```python
from build123d import *

# Parameters (mm, degrees)
SKETCH1_R                = 59
EXTRUDE1_DEPTH           = 3
EXTRUDE2_DEPTH           = 3
CIRPATTERN1_COUNT        = 6
F_2_0_2_DIAMETER_HOLE1_D = 2
F_2_0_2_DIAMETER_HOLE3_D = 2
CIRPATTERN2_COUNT        = 6


with BuildPart() as part:
    # Sketch1 → Extrude1 (new, symmetric)
    with BuildSketch(Plane(origin=(0, 0, 0), x_dir=(0, 0, -1), z_dir=(1, 0, 0))):
        Circle(SKETCH1_R)
        Polygon((23.694176429, 16.590840947), (-2.521001516, 28.815179183), (-26.215177945, 12.224338236), (-23.694176429, -16.590840947), (2.521001516, -28.815179183), (26.215177945, -12.224338236), align=None, mode=Mode.SUBTRACT)
    extrude(amount=EXTRUDE1_DEPTH, both=True)

    # Sketch2 → Extrude2 (add, symmetric)
    with BuildSketch(Plane(origin=(0, 0, 0), x_dir=(0, 0, -1), z_dir=(1, 0, 0))):
        with BuildLine():
            Line((-2, 67.961805723), (-0.262709442, 61.478149092))
            ThreePointArc((-0.262709442, 61.478149092), (-0.58620663, 59.77173183), (-2.122608272, 58.961805723))
            ThreePointArc((-2.122608272, 58.961805723), (28.679663449, 51.560419941), (51.21368579, 29.294340542))
            ThreePointArc((51.21368579, 29.294340542), (36.791707484, 48.186627241), (17.927108603, 62.644803614))
            ThreePointArc((17.927108603, 62.644803614), (8.312130826, 66.609702921), (-2, 67.961805723))
        make_face()
    extrude2 = extrude(amount=EXTRUDE2_DEPTH, both=True)

    # CirPattern1: Extrude2 ×6 about axis
    cirpattern1_axis = Axis((0, 0, 0), (1, 0, 0))
    for i in range(1, CIRPATTERN1_COUNT):
        add(extrude2.rotate(cirpattern1_axis, i * 360 / CIRPATTERN1_COUNT))

    # Ø2.0 (2) Diameter Hole1 (through all)
    with Locations(Plane(origin=(3, 0, 0), x_dir=(0, 0, -1), z_dir=(1, 0, 0))):
        with Locations((-2.521001516, 28.815179183), (23.694176429, 16.590840947), (26.215177945, -12.224338236), (2.521001516, -28.815179183), (-23.694176429, -16.590840947), (-26.215177945, 12.224338236)):
            Hole(F_2_0_2_DIAMETER_HOLE1_D / 2)

    # Ø2.0 (2) Diameter Hole3 (through all)
    with Locations(Plane(origin=(3, 0, 0), x_dir=(0, 0, -1), z_dir=(1, 0, 0))):
        with Locations((6.519493728, 24.599527017)):
            f_2_0_2_diameter_hole3 = Hole(F_2_0_2_DIAMETER_HOLE3_D / 2)

    # CirPattern2: Ø2.0 (2) Diameter Hole3 ×6 about axis
    cirpattern2_axis = Axis((0, 0, 0), (1, 0, 0))
    for i in range(1, CIRPATTERN2_COUNT):
        add(f_2_0_2_diameter_hole3.rotate(cirpattern2_axis, i * 360 / CIRPATTERN2_COUNT), mode=Mode.SUBTRACT)


solid = part.part
```
Here's how the part is built. I have some questions about the finished solid (model axes, mm). A direction names the side the tool comes from. Round coordinates to 2 decimals unless told otherwise and drop trailing zeros. Order: outer loops, then holes, each group sorted by start corner. A loop starts at its lowest first (then second) coordinate and runs counter-clockwise, first axis right, second up. Notation, with made-up numbers: (23.5, 56) -> (50.5, 56) arc R26 cw to (50.5, 85) -> close; hole circle Ø5 at (16.25, 48.5). An arc over 180 degrees is marked (long way). Use a Markdown table: item, result. Add a question column.
(1) If we mould it in two halves opening along Y, with no side actions, what happens to faces 1 (the face through (-3, 26, 14)), 2 (the face through (0.042, -48.714, 36.261)), 3 (the face through (0.042, -26.684, 2.05))? For each: released by +Y, released by -Y, zero draft, split by the parting line, or undercut.
(2) Suppose I cut it at B-B, the plane y = 2.5. Please give me the cut outline in (x, z), and give its area (3 significant figures).
(3) Suppose I cut it at D-D, the plane z = -48.5. Please give me the cut outline in (x, y), and give its area (3 significant figures).
(4) Suppose I cut it at C-C, the plane y = 39. Please give me the cut outline in (x, z).
(5) I need wall thicknesses on line 1 along Z through (x, y) = (-2, 6); line 2 along Y through (x, z) = (-0.8, 54); line 3 along Z through (x, y) = (1.25, 15). Which ranges of each line are inside material? Lowest first, please.
(6) For pin 1 Ø3 at (x, z) = (-2, -31.5) entering from +Y; pin 2 Ø1.2 at (y, z) = (-12.22, -26.22) entering from +X; pin 3 Ø1.5 at (x, y) = (1.5, 9.5) entering from -Z; pin 4 Ø2 at (x, z) = (1, 44.5) entering from -Y, each with a flat end and sliding along its axis, tell me the tip position at first contact or that it passes through.
(7) For faces 4 (the face through (0.042, -33.373, 55.517)), 5 (the face through (0.042, 23.449, 10.185)), 6 (the face through (0.042, -64.765, -1.144)), which set-ups out of +Z, -Z, +X, -X, +Y, -Y let a thin tool reach every point of the face, with its end or its side?
(8) Suppose I cut it at A-A, the plane z = -9.5. Please give me the cut outline in (x, y).
Verdict:
| question | item | result |
|---|---|---|
| 1 | face 1 | zero draft |
| 1 | face 2 | released by -Y |
| 1 | face 3 | undercut |
| 2 | outline | (-3, -62.26) -> (3, -62.26) -> (3, -24.93) -> (-3, -24.93) -> close; (-3, 25.36) -> (3, 25.36) -> (3, 61.38) -> (-3, 61.38) -> close |
| 2 | area | 440 mm2 |
| 3 | outline | (-3, -44.77) -> (3, -44.77) -> (3, 33.74) -> (-3, 33.74) -> close |
| 3 | area | 471 mm2 |
| 4 | outline | (-3, -44.8) -> (3, -44.8) -> (3, 54.95) -> (-3, 54.95) -> close |
| 5 | line 1 | -62.7 to -25.32, 25.67 to 60.58 |
| 5 | line 2 | -31.86 to 24.06, 30.68 to 40.02 |
| 5 | line 3 | -63.21 to -23.83, 22.25 to 57.85 |
| 6 | pin 1 | y = 54.33 |
| 6 | pin 2 | through |
| 6 | pin 3 | z = -63.06 |
| 6 | pin 4 | y = -40.67 |
| 7 | face 4 | +X, -X, -Y |
| 7 | face 5 | +X, -X |
| 7 | face 6 | -Z, +X, -X |
| 8 | outline | (-3, -58.51) -> (3, -58.51) -> (3, -23.93) -> (-3, -23.93) -> close; (-3, 23.21) -> (3, 23.21) -> (3, 66.27) -> (-3, 66.27) -> close |
